The drawing under review shows one solid part. Ordinate dimensions are in mm from its lowest x, y, z. A direction names the side the tool comes from. Give positions to 0.01 mm unless a question says otherwise; leave off trailing zeros. Loops run counter-clockwise (first coordinate to the right, second up) from the corner with the lowest first, then second, coordinate; pieces in that order, holes last. Notation, with made-up numbers: M 89,-11.5 L 148,-11.5 A32 ccw 148,24.5 Z; hole C -13.75,-39 d3. An arc over 180 degrees is marked long. One line per item, written item: value. Start each with the question number.
Q1. To check wall thickness, follow line 1 along X through (y, z) = (5, 20); line 2 along Z through (x, y) = (25, 1); line 3 along X through (y, z) = (1.75, 29.5). State the ranges of each line that lie inside material, in increasing order. Write a range as from..to.
Q2. For pin 1 (4.5 mm diameter, centred on x = 11.56, z = 6.56, fed in from -Y); pin 2 (6.5 mm diameter, centred on x = 11.56, z = 33.44, fed in from +Y); pin 3 (4 mm diameter, centred on x = 38, y = 7, fed in from +Z); pin 4 (3 mm diameter, centred on y = 4.5, z = 13, fed in from +X) (3 decimals), all flat-tipped, find the tip position at first contact; note any pin that passes through.
Q3. Mouldability with a two-part tool opening along Z and no side actions: class the marked faces 1, 2 and 3 as released by +Z, released by -Z, zero draft, split by the parting line, or undercut.
Q4. We need section A-A on z = 20. Write out the cut boundary in (x, y).
Q5. For the marked faces 4 and 5, list the 3-axis set-ups (+Z, -Z, +X, -X, +Y, -Y) from which the entire face can be reached by the end or side of a thin tool; tool diameter is ignored.
Q6. We need section D-D on z = 35.5. Write out the cut boundary in (x, y), plus the area to 3 significant figures.
Q7. We need section C-C on y = 4.75. Write out the cut boundary in (x, z).
Q8. We need section B-B on x = 20. Write out the cut boundary in (y, z).
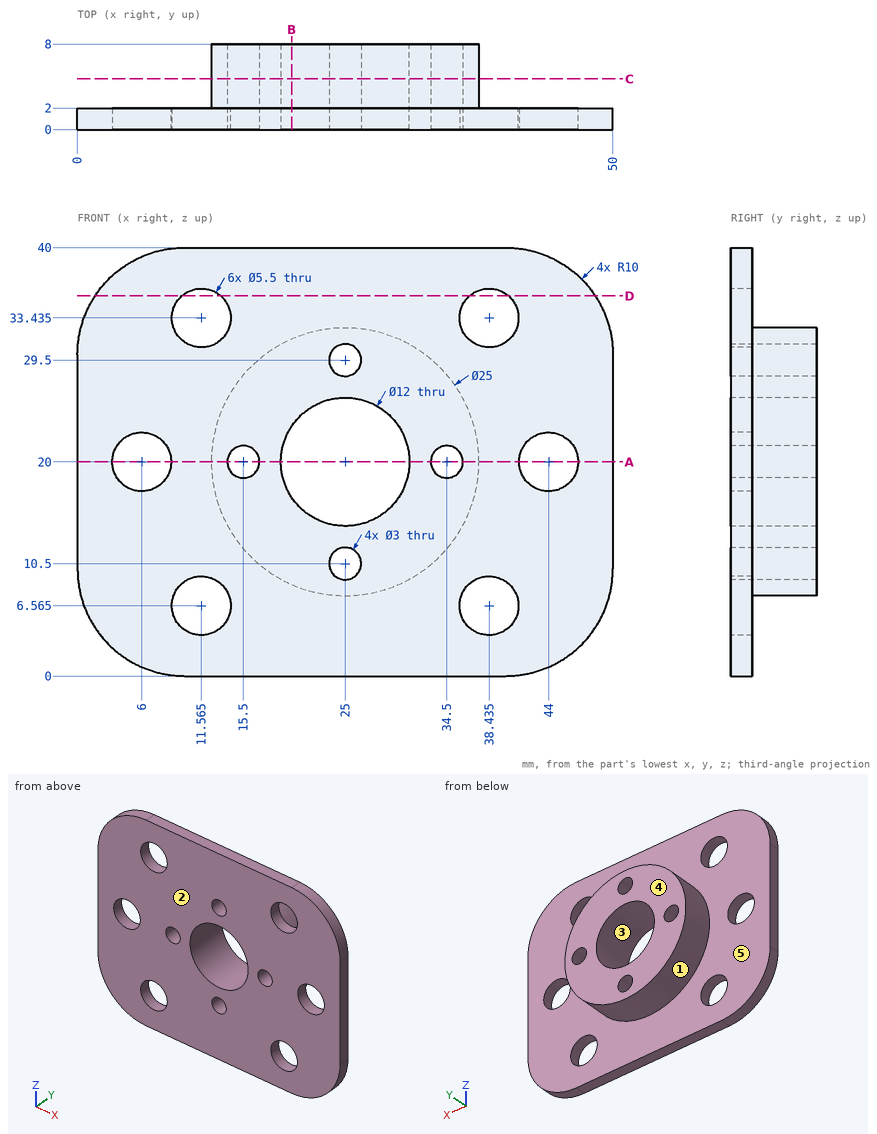
Solved:
1. line 1: 12.5..14, 17..19, 31..33, 36..37.5
1. line 2: 0..9, 12..14, 26..28, 31..40
1. line 3: 0..23.5, 26.5..50
2. pin 1: through
2. pin 2: y = 2
2. pin 3: z = 25.94
2. pin 4: x = 36.225
3. face 1: split by the parting line
3. face 2: zero draft
3. face 3: undercut
4. outline: M 0,0 L 3.25,0 L 3.25,2 L 0,2 Z; M 8.75,0 L 14,0 L 14,8 L 12.5,8 L 12.5,2 L 8.75,2 Z; M 17,0 L 19,0 L 19,8 L 17,8 Z; M 31,0 L 33,0 L 33,8 L 31,8 Z; M 36,0 L 41.25,0 L 41.25,2 L 37.5,2 L 37.5,8 L 36,8 Z; M 46.75,0 L 50,0 L 50,2 L 46.75,2 Z
5. face 4: +Z, -Z, +X, -X, +Y
5. face 5: +Y
6. outline: M 1.65,0 L 9.75,0 L 9.75,2 L 1.65,2 Z; M 13.38,0 L 36.62,0 L 36.62,2 L 13.38,2 Z; M 40.25,0 L 48.35,0 L 48.35,2 L 40.25,2 Z
6. area: 78.9 mm2
7. outline: C 25,20 d25; hole C 15.5,20 d3; hole C 25,20 d12; hole C 25,10.5 d3; hole C 25,29.5 d3; hole C 34.5,20 d3
8. outline: M 0,0 L 2,0 L 2,8.54 L 8,8.54 L 8,16.68 L 0,16.68 Z; M 0,23.32 L 8,23.32 L 8,31.46 L 2,31.46 L 2,40 L 0,40 Z
